Work out the finished part from the listing and answer in its coordinate system (mm). Coordinates: 2 decimals unless noted, no trailing zeros. Loops run counter-clockwise (first coordinate to the right, second up) from the corner with the lowest first, then second, coordinate; pieces in that order, holes last. Notation, with made-up numbers: (-31.75, -26.75) - (-9.75, -26.75) arc R8 ccw to (-9.75, -22.75) - close; hole circle Ø1 at (-39, -14). An arc over 180 degrees is marked (long way). Write each question's results on one line, items separated by ' | '. Start each with the question number.
1. Find the intervals of material crossed by line 1 along Y through (x, z) = (-34.5, 2.25); line 2 along Y through (x, z) = (-41, 2.2); line 3 along X through (y, z) = (105, 4.65), in increasing order. Write a range as [from, to].
2. A cutting plane is placed at C-C on z = 3.05. State how many separate pieces and enclosed holes the cut face has, then the cut area to 3 significant figures.
3. A cutting plane is placed at D-D on y = 11. Determine the outline of the cut face in (x, z), then the cut area to 3 significant figures.
4. Determine the mould class of faces 1 (the flat face through (-80, 40, 5)), 2 (the cylindrical face through (-215.522, 99.513, 2.465)), 3 (the cylindrical face through (-284.01, -49.21, 2.46)) for opening direction X: released by +X, released by -X, zero draft, split by the parting line, or undercut.
5. A cutting plane is placed at A-A on x = -78. Determine the outline of the cut face in (y, z), then the cut area to 3 significant figures.
6. A cutting plane is placed at B-B on y = 135. Determine the outline of the cut face in (x, z).
from build123d import *

# Parameters (mm, degrees)
F0_R     = 40
F0_W     = 50
F0_H     = 5
F0_W_2   = 105
F1_DEPTH = 5


with BuildPart() as f1:
    # F0 (on Top) → F1 (new body)
    with BuildSketch(Plane.XY):
        with BuildLine():
            ThreePointArc((146.020335, 147.5), (130.643441, 184.623106), (93.520335, 200))
            Line((93.520335, 200), (-246.479665, 200))
            ThreePointArc((-246.479665, 200), (-283.602771, 184.623106), (-298.979665, 147.5))
            Line((-298.979665, 147.5), (-298.979665, -12.5))
            ThreePointArc((-298.979665, -12.5), (-283.602771, -49.623106), (-246.479665, -65))
            Line((-246.479665, -65), (93.520335, -65))
            ThreePointArc((93.520335, -65), (130.643441, -49.623106), (146.020335, -12.5))
            Line((146.020335, -12.5), (146.020335, 65))
            Line((146.020335, 65), (146.020335, 70))
            Line((146.020335, 70), (146.020335, 147.5))
        make_face()
        with Locations((-233.979665, 0)):
            Circle(F0_R, mode=Mode.SUBTRACT)
        with Locations((-128.979665, 0)):
            Circle(F0_R, mode=Mode.SUBTRACT)
        with Locations((-23.979665, 0)):
            Circle(F0_R, mode=Mode.SUBTRACT)
        with Locations((81.020335, 0)):
            Circle(F0_R, mode=Mode.SUBTRACT)
        with Locations((-233.979665, 67.5)):
            Rectangle(F0_W, F0_H, mode=Mode.SUBTRACT)
        with Locations((-233.979665, 135)):
            Circle(F0_R, mode=Mode.SUBTRACT)
        with Locations((-128.979665, 135)):
            Circle(F0_R, mode=Mode.SUBTRACT)
        with Locations((-76.479665, 67.5)):
            Rectangle(F0_W_2, F0_H, mode=Mode.SUBTRACT)
        with Locations((81.020335, 67.5)):
            Rectangle(F0_W, F0_H, mode=Mode.SUBTRACT)
        with Locations((-23.979665, 135)):
            Circle(F0_R, mode=Mode.SUBTRACT)
        with Locations((81.020335, 135)):
            Circle(F0_R, mode=Mode.SUBTRACT)
    extrude(amount=F1_DEPTH)


solid = f1.part
Values:
1) line 1: [-65, -38.59], [38.59, 65], [70, 96.41], [173.59, 200] | line 2: [-65, -36.2], [36.2, 65], [70, 98.8], [171.2, 200] | line 3: [-298.98, -260.44], [-207.52, -155.44], [-102.52, -50.44], [2.48, 54.56], [107.48, 146.02]
2) separate pieces: 1 | enclosed holes: 11 | area: 74,300 mm^2
3) outline: (-298.98, 0) - (-272.44, 0) - (-272.44, 5) - (-298.98, 5) - close; (-195.52, 0) - (-167.44, 0) - (-167.44, 5) - (-195.52, 5) - close; (-90.52, 0) - (-62.44, 0) - (-62.44, 5) - (-90.52, 5) - close; (14.48, 0) - (42.56, 0) - (42.56, 5) - (14.48, 5) - close; (119.48, 0) - (146.02, 0) - (146.02, 5) - (119.48, 5) - close | area: 687 mm^2
4) face 1: zero draft | face 2: undercut | face 3: released by -X
5) outline: (-65, 0) - (65, 0) - (65, 5) - (-65, 5) - close; (70, 0) - (200, 0) - (200, 5) - (70, 5) - close | area: 1,300 mm^2
6) outline: (-298.98, 0) - (-273.98, 0) - (-273.98, 5) - (-298.98, 5) - close; (-193.98, 0) - (-168.98, 0) - (-168.98, 5) - (-193.98, 5) - close; (-88.98, 0) - (-63.98, 0) - (-63.98, 5) - (-88.98, 5) - close; (16.02, 0) - (41.02, 0) - (41.02, 5) - (16.02, 5) - close; (121.02, 0) - (146.02, 0) - (146.02, 5) - (121.02, 5) - close
